Here's how the part is built. I have some questions about the finished solid (model axes, mm). Face numbers are marked on the shaded views. A direction names the side the tool comes from. Coordinates: 2 decimals unless noted, no trailing zeros. Loops run counter-clockwise (first coordinate to the right, second up) from the corner with the lowest first, then second, coordinate; pieces in that order, holes last. Notation, with made-up numbers: (-18, -31.5) - (33, -31.5) arc R22 ccw to (33, 2.5) - close; hole circle Ø4 at (-14, 53). An arc over 180 degrees is marked (long way). Use a Markdown table: item, result.
Autodesk Inventor part; units mm, degrees
ref_plane "YZ Plane" through (0, 0, 0) normal (1, 0, 0) x (0, 1, 0)
ref_plane "XZ Plane" through (0, 0, 0) normal (0, 1, 0) x (-1, 0, 0)
ref_plane "XY Plane" through (0, 0, 0) normal (0, 0, 1) x (1, 0, 0)
sketch "Sketch4" plane through (0, 0, 0) normal (0, 0, 1) x (1, 0, 0)
  line L0 (0, 0) -> (-60, 0)
  line L1 (-60, 0) -> (-60, 20)
  line L2 (-60, 20) -> (0, 20)
  line L3 (0, 20) -> (0, 0)
  dimension "d37" = 60
  dimension "d38" = 20
extrude "Extrusion2" add sketch "Sketch4" along normal blind 10
hole "Hole2" at (-30, 10, 10) direction (0, 0, -1) diameter 6.5 depth 10 tip angle 118 counterbore diameter 10.5 counterbore depth 6.5
hole "Hole3" at (-55, 15, 10) direction (0, 0, -1) diameter 5.5 depth 10 tip angle 118 counterbore diameter 9 counterbore depth 8
hole "Hole4" at (-5, 15, 10) direction (0, 0, -1) diameter 5.5 depth 10 tip angle 118 counterbore diameter 9 counterbore depth 8
hole "Hole5" at (-5, 5, 10) direction (0, 0, -1) diameter 5.5 depth 10 tip angle 118 counterbore diameter 9 counterbore depth 8
hole "Hole6" at (-55, 5, 10) direction (0, 0, -1) diameter 5.5 depth 10 tip angle 118 counterbore diameter 9 counterbore depth 8
properties part number "GARFO" material "Aluminium AW-7020"
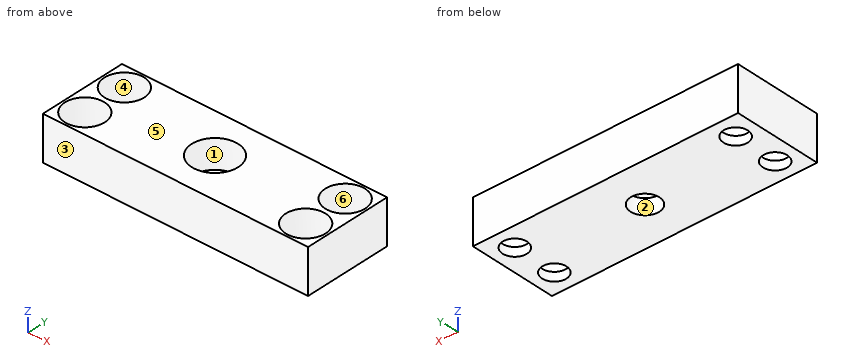
Q1. I want a section at A-A, the plane x = -5. Write out the boundary of the cut face in (y, z).
Check values:
| item | result |
|---|---|
| outline | (0, 0) - (2.25, 0) - (2.25, 2) - (0.5, 2) - (0.5, 10) - (0, 10) - close; (7.75, 0) - (12.25, 0) - (12.25, 2) - (10.5, 2) - (10.5, 10) - (9.5, 10) - (9.5, 2) - (7.75, 2) - close; (17.75, 0) - (20, 0) - (20, 10) - (19.5, 10) - (19.5, 2) - (17.75, 2) - close |
Q2. I want a section at C-C, the plane y = 11.25. Write out the boundary of the cut face in (x, z), then the cut area to 3 significant figures.
Check values:
| item | result |
|---|---|
| outline | (-60, 0) - (-33, 0) - (-33, 3.5) - (-35.1, 3.5) - (-35.1, 10) - (-52.51, 10) - (-52.51, 2) - (-57.49, 2) - (-57.49, 10) - (-60, 10) - close; (-27, 0) - (0, 0) - (0, 10) - (-2.51, 10) - (-2.51, 2) - (-7.49, 2) - (-7.49, 10) - (-24.9, 10) - (-24.9, 3.5) - (-27, 3.5) - close |
| area | 433 mm^2 |
Q3. Please list where these lines run through material, in increasing order: L1, parallel to X at y = 5, z = 0.45; L2, parallel to Y at x = -55, z = 5.75; L3, parallel to Y at x = -53, z = 7.5. Write a range as from..to.
Check values:
| item | result |
|---|---|
| L1 | -60..-57.75, -52.25..-7.75, -2.25..0 |
| L2 | 0..0.5, 9.5..10.5, 19.5..20 |
| L3 | 0..0.97, 9.03..10.97, 19.03..20 |
Q4. If we mould it in two halves opening along Y, with no side actions, what happens to the marked faces 3, 4, 5 and 6? For each: pulls with the +Y half, pulls with the -Y half, needs draft (parallel to the pull), parting line crosses it, or undercut.
Check values:
| item | result |
|---|---|
| face 3 | pulls with the -Y half |
| face 4 | undercut |
| face 5 | needs draft |
| face 6 | undercut |
Q5. Which directions (+Z, -Z, +X, -X, +Y, -Y) give clear straight access to the entire face, cutting with the end or side of a thin tool? Please do the marked faces 1 and 2.
Check values:
| item | result |
|---|---|
| face 1 | +Z |
| face 2 | +Z, -Z |
Q6. I want a section at D-D, the plane y = 18.5. Write out the boundary of the cut face in (x, z), then the cut area to 3 significant figures.
Check values:
| item | result |
|---|---|
| outline | (-60, 0) - (0, 0) - (0, 10) - (-2.17, 10) - (-2.17, 2) - (-7.83, 2) - (-7.83, 10) - (-52.17, 10) - (-52.17, 2) - (-57.83, 2) - (-57.83, 10) - (-60, 10) - close |
| area | 509 mm^2 |
Q7. Will these pins go through, and if not, where does the flat tip stop? P1, Ø5, axis at x = -30, y = 10, coming from the -Z side; P2, Ø7, axis at x = -54.5, y = 17, coming from the +Z side.
Check values:
| item | result |
|---|---|
| P1 | through |
| P2 | z = 10 |
Q8. I want a section at B-B, the plane z = 8.5. Write out the boundary of the cut face in (x, y), then the cut area to 3 significant figures.
Check values:
| item | result |
|---|---|
| outline | (-60, 0) - (0, 0) - (0, 20) - (-60, 20) - close; hole circle Ø9 at (-55, 5); hole circle Ø9 at (-55, 15); hole circle Ø10.5 at (-30, 10); hole circle Ø9 at (-5, 5); hole circle Ø9 at (-5, 15) |
| area | 859 mm^2 |
